The listing builds one solid part. Answer for the finished solid, in the listing's coordinates (mm). Face numbers are marked on the shaded views. A direction names the side the tool comes from. Coordinates: 2 decimals unless noted, no trailing zeros. Order: outer loops, then holes, each group sorted by start corner. A loop starts at its lowest first (then second) coordinate and runs counter-clockwise, first axis right, second up. Notation, with made-up numbers: (8.5, 52) -> (37.5, 52) arc R31 ccw to (37.5, 89) -> close; hole circle Ø11 at (-37, 82). An arc over 180 degrees is marked (long way). Answer in a Markdown table with one row per item.
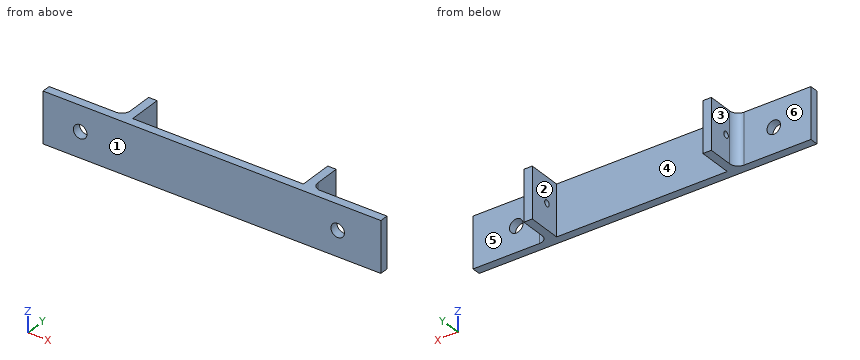
```python
from build123d import *

# Parameters (mm, degrees)
SKETCH1_W           = 200
SKETCH1_H           = 30
BOSS_EXTRUDE1_DEPTH = 5
SKETCH2_W           = 5
SKETCH2_H           = 30
BOSS_EXTRUDE2_DEPTH = 20
FILLET1_R           = 5
SKETCH3_R           = 1.85
CUT_EXTRUDE2_DEPTH  = 159.209512988
SKETCH4_R           = 4
CUT_EXTRUDE3_DEPTH  = 104.07764064
SKETCH5_R           = 4
CUT_EXTRUDE4_DEPTH  = 104.07764064


with BuildPart() as part:
    # Sketch1 → Boss-Extrude1 (new body)
    with BuildSketch(Plane(origin=(0, 0, 0), x_dir=(1, 0, 0), z_dir=(0, 1, 0))):
        Rectangle(SKETCH1_W, SKETCH1_H)
    extrude(amount=BOSS_EXTRUDE1_DEPTH)

    # Sketch2 → Boss-Extrude2 (add)
    with BuildSketch(Plane(origin=(0, 5, 0), x_dir=(1, 0, 0), z_dir=(0, 1, 0))):
        with Locations((-53, 0)):
            Rectangle(SKETCH2_W, SKETCH2_H)
        with Locations((53, 0)):
            Rectangle(SKETCH2_W, SKETCH2_H)
    extrude(amount=BOSS_EXTRUDE2_DEPTH)

    # Fillet1
    fillet1_edges = [part.edges().sort_by_distance(p)[0] for p in [
        (-55.5, 5, 0),
        (55.5, 5, 0),
    ]]
    fillet(fillet1_edges, radius=FILLET1_R)

    # Sketch3 → Cut-Extrude2 (cut, through all)
    with BuildSketch(Plane.ZY.offset(55.5)):
        with Locations((0, 12.94)):
            Circle(SKETCH3_R)
    extrude(amount=-CUT_EXTRUDE2_DEPTH, mode=Mode.SUBTRACT)

    # Sketch4 → Cut-Extrude3 (cut, through all)
    with BuildSketch(Plane(origin=(0, 5, 0), x_dir=(1, 0, 0), z_dir=(0, 1, 0))):
        with Locations(Location((-78, 0, 0), (0, 0, 270))):
            Circle(SKETCH4_R)
    extrude(amount=-CUT_EXTRUDE3_DEPTH, mode=Mode.SUBTRACT)

    # Sketch5 → Cut-Extrude4 (cut, through all)
    with BuildSketch(Plane(origin=(0, 5, 0), x_dir=(1, 0, 0), z_dir=(0, 1, 0))):
        with Locations(Location((74.4, 0, 0), (0, 0, 270))):
            Circle(SKETCH5_R)
    extrude(amount=-CUT_EXTRUDE4_DEPTH, mode=Mode.SUBTRACT)


solid = part.part
```
(1) Flat-ended cylindrical pins translate along their axes: pin 1 (6 mm diameter, centred on y = 12.94, z = 0, fed in from +X); pin 2 (6 mm diameter, centred on y = 15.5, z = 3, fed in from -X); pin 3 (9 mm diameter, centred on x = 77, z = -6.5, fed in from +Y). Find the tip coordinate at first contact, or state that the pin passes through.
Check values:
| item | result |
|---|---|
| pin 1 | x = 55.5 |
| pin 2 | x = -55.5 |
| pin 3 | y = 5 |
(2) Which of the six approach directions +Z, -Z, +X, -X, +Y, -Y give full straight-line access (tool end or side, diameter ignored) to the marked faces 4, 5 and 6?
Check values:
| item | result |
|---|---|
| face 4 | +Z, -Z, +Y |
| face 5 | +Z, -Z, +X, +Y |
| face 6 | +Z, -Z, -X, +Y |
(3) A cutting plane is placed at C-C, the plane z = 0. Count the separate pieces of the cut face and the enclosed holes in it, then the cut area to 3 significant figures.
Check values:
| item | result |
|---|---|
| separate pieces | 5 |
| enclosed holes | 0 |
| area | 1,090 mm² |
(4) For a pull along X with two mould halves and no side action, classify the marked faces 1, 2 and 3 as released by +X, released by -X, zero draft, split by the parting line, or undercut.
Check values:
| item | result |
|---|---|
| face 1 | zero draft |
| face 2 | undercut |
| face 3 | released by -X |
(5) A cutting plane is placed at B-B, the plane y = 16.75. Determine the outline of the cut face in (x, z), then the cut area to 3 significant figures.
Check values:
| item | result |
|---|---|
| outline | (-55.5, -15) -> (-50.5, -15) -> (-50.5, 15) -> (-55.5, 15) -> close; (50.5, -15) -> (55.5, -15) -> (55.5, 15) -> (50.5, 15) -> close |
| area | 300 mm² |
(6) A cutting plane is placed at A-A, the plane x = 74.4. Determine the outline of the cut face in (y, z).
Check values:
| item | result |
|---|---|
| outline | (0, -15) -> (5, -15) -> (5, -4) -> (0, -4) -> close; (0, 4) -> (5, 4) -> (5, 15) -> (0, 15) -> close |
(7) Find the intervals of material crossed by line 1 along X through (y, z) = (3.4, 0); line 2 along X through (y, z) = (15.25, -10.75); line 3 along Y through (x, z) = (-53.65, 0), in increasing order. Write a range as from..to.
Check values:
| item | result |
|---|---|
| line 1 | -100..-82, -74..70.4, 78.4..100 |
| line 2 | -55.5..-50.5, 50.5..55.5 |
| line 3 | 0..11.09, 14.79..25 |
(8) A cutting plane is placed at D-D, the plane z = -13. Determine the outline of the cut face in (x, y), then the cut area to 3 significant figures.
Check values:
| item | result |
|---|---|
| outline | (-100, 0) -> (100, 0) -> (100, 5) -> (60.5, 5) arc R5 cw to (55.5, 10) -> (55.5, 25) -> (50.5, 25) -> (50.5, 5) -> (-50.5, 5) -> (-50.5, 25) -> (-55.5, 25) -> (-55.5, 10) arc R5 cw to (-60.5, 5) -> (-100, 5) -> close |
| area | 1,210 mm² |
